```python
from build123d import *

# Parameters (mm, degrees)
F1_DEPTH     = 6
F2_C1_SIZE2  = 3
F2_C1_SIZE   = 1.7320508076
F2_C2_SIZE2  = 3
F2_C2_SIZE   = 1.7320508076
F2_C3_SIZE2  = 1.7320508076
F2_C3_SIZE   = 3
F2_C4_SIZE2  = 3
F2_C4_SIZE   = 1.7320508076
F2_C5_SIZE2  = 1.7320508076
F2_C5_SIZE   = 3
F2_C6_SIZE2  = 3
F2_C6_SIZE   = 1.7320508076
F2_C7_SIZE2  = 1.7320508076
F2_C7_SIZE   = 3
F2_C8_SIZE2  = 3
F2_C8_SIZE   = 1.7320508076
F2_C9_SIZE2  = 1.7320508076
F2_C9_SIZE   = 3
F2_C10_SIZE2 = 3
F2_C10_SIZE  = 1.7320508076
F2_C11_SIZE2 = 3
F2_C11_SIZE  = 1.7320508076
F2_C12_SIZE2 = 3
F2_C12_SIZE  = 1.7320508076
F2_C13_SIZE2 = 1.7320508076
F2_C13_SIZE  = 3
F2_C14_SIZE2 = 3
F2_C14_SIZE  = 1.7320508076
F2_C15_SIZE2 = 3
F2_C15_SIZE  = 1.7320508076
F2_C16_SIZE2 = 3
F2_C16_SIZE  = 1.7320508076
F2_C17_SIZE2 = 1.7320508076
F2_C17_SIZE  = 3
F2_C18_SIZE2 = 3
F2_C18_SIZE  = 1.7320508076
F2_C19_SIZE2 = 3
F2_C19_SIZE  = 1.7320508076
F2_C20_SIZE2 = 3
F2_C20_SIZE  = 1.7320508076
F2_C21_SIZE2 = 1.7320508076
F2_C21_SIZE  = 3
F2_C22_SIZE2 = 3
F2_C22_SIZE  = 1.7320508076
F2_C23_SIZE2 = 3
F2_C23_SIZE  = 1.7320508076
F2_C24_SIZE2 = 3
F2_C24_SIZE  = 1.7320508076
F3_R         = 1


with BuildPart() as f1:
    # F0 (on Top) → F1 (new body)
    with BuildSketch(Plane.XY):
        with BuildLine():
            ThreePointArc((5.4975, 9.5219493146), (9.5219493146, 5.4975), (10.995, 0))
            Line((10.995, 0), (14.995, 0))
            ThreePointArc((14.995, 0), (17.8875950663, 4.5341861944), (23.2185377782, 3.8221465425))
            Line((23.2185377782, 3.8221465425), (38.9711431703, 22.5))
            Line((38.9711431703, 22.5), (14.9193448919, 18.1967702834))
            ThreePointArc((14.9193448919, 18.1967702834), (12.870517963, 13.2240186428), (7.4975, 12.9860509297))
            Line((7.4975, 12.9860509297), (5.4975, 9.5219493146))
        make_face()
        with BuildLine():
            ThreePointArc((-5.4975, 9.5219493146), (0, 10.995), (5.4975, 9.5219493146))
            Line((5.4975, 9.5219493146), (7.4975, 12.9860509297))
            ThreePointArc((7.4975, 12.9860509297), (5.0170771033, 17.7582048372), (8.2991928863, 22.0189168259))
            Line((8.2991928863, 22.0189168259), (0, 45))
            Line((0, 45), (-8.2991928863, 22.0189168259))
            ThreePointArc((-8.2991928863, 22.0189168259), (-5.0170771033, 17.7582048372), (-7.4975, 12.9860509297))
            Line((-7.4975, 12.9860509297), (-5.4975, 9.5219493146))
        make_face()
        with BuildLine():
            ThreePointArc((-10.995, 0), (-9.5219493146, 5.4975), (-5.4975, 9.5219493146))
            Line((-5.4975, 9.5219493146), (-7.4975, 12.9860509297))
            ThreePointArc((-7.4975, 12.9860509297), (-12.870517963, 13.2240186428), (-14.9193448919, 18.1967702834))
            Line((-14.9193448919, 18.1967702834), (-38.9711431703, 22.5))
            Line((-38.9711431703, 22.5), (-23.2185377782, 3.8221465425))
            ThreePointArc((-23.2185377782, 3.8221465425), (-17.8875950663, 4.5341861944), (-14.995, 0))
            Line((-14.995, 0), (-10.995, 0))
        make_face()
        with BuildLine():
            Line((-7.4975, -12.9860509297), (-5.4975, -9.5219493146))
            ThreePointArc((-5.4975, -9.5219493146), (-9.5219493146, -5.4975), (-10.995, 0))
            Line((-10.995, 0), (-14.995, 0))
            ThreePointArc((-14.995, 0), (-17.8875950663, -4.5341861944), (-23.2185377782, -3.8221465425))
            Line((-23.2185377782, -3.8221465425), (-38.9711431703, -22.5))
            Line((-38.9711431703, -22.5), (-14.9193448919, -18.1967702834))
            ThreePointArc((-14.9193448919, -18.1967702834), (-12.870517963, -13.2240186428), (-7.4975, -12.9860509297))
        make_face()
        with BuildLine():
            Line((7.4975, -12.9860509297), (5.4975, -9.5219493146))
            ThreePointArc((5.4975, -9.5219493146), (0, -10.995), (-5.4975, -9.5219493146))
            Line((-5.4975, -9.5219493146), (-7.4975, -12.9860509297))
            ThreePointArc((-7.4975, -12.9860509297), (-5.0170771033, -17.7582048372), (-8.2991928863, -22.0189168259))
            Line((-8.2991928863, -22.0189168259), (0, -45))
            Line((0, -45), (8.2991928863, -22.0189168259))
            ThreePointArc((8.2991928863, -22.0189168259), (5.0170771033, -17.7582048372), (7.4975, -12.9860509297))
        make_face()
        with BuildLine():
            Line((14.995, 0), (10.995, 0))
            ThreePointArc((10.995, 0), (9.5219493146, -5.4975), (5.4975, -9.5219493146))
            Line((5.4975, -9.5219493146), (7.4975, -12.9860509297))
            ThreePointArc((7.4975, -12.9860509297), (12.870517963, -13.2240186428), (14.9193448919, -18.1967702834))
            Line((14.9193448919, -18.1967702834), (38.9711431703, -22.5))
            Line((38.9711431703, -22.5), (23.2185377782, -3.8221465425))
            ThreePointArc((23.2185377782, -3.8221465425), (17.8875950663, -4.5341861944), (14.995, 0))
        make_face()
    extrude(amount=F1_DEPTH)

    # F2: chamfer of 3 x 1.7320508076 on 24 edges, made by hand

    # F2_c1
    f2_c1_edges = [f1.edges().sort_by_distance(p)[0] for p in [
        (31.0948404742, 13.1610732713, 0),
    ]]
    f2_c1_side = f1.faces().sort_by_distance((31.0948404742, 13.1610732713, 0.0346410162))[0]
    chamfer(f2_c1_edges, length=F2_C1_SIZE, length2=F2_C1_SIZE2, reference=f2_c1_side)

    # F2_c2
    f2_c2_edges = [f1.edges().sort_by_distance(p)[0] for p in [
        (31.0948404742, 13.1610732713, 6),
    ]]
    f2_c2_side = f1.faces().sort_by_distance((31.0948404742, 13.1610732713, 5.9653589838))[0]
    chamfer(f2_c2_edges, length=F2_C2_SIZE, length2=F2_C2_SIZE2, reference=f2_c2_side)

    # F2_c3
    f2_c3_edges = [f1.edges().sort_by_distance(p)[0] for p in [
        (24.6342857936, 19.9349198346, 0),
    ]]
    f2_c3_side = f1.faces().sort_by_distance((24.6342857936, 19.9349198346, 0.0346410162))[0]
    chamfer(f2_c3_edges, length=F2_C3_SIZE, length2=F2_C3_SIZE2, reference=f2_c3_side)

    # F2_c4
    f2_c4_edges = [f1.edges().sort_by_distance(p)[0] for p in [
        (24.6342857936, 19.9349198346, 6),
    ]]
    f2_c4_side = f1.faces().sort_by_distance((24.6342857936, 19.9349198346, 5.9653589838))[0]
    chamfer(f2_c4_edges, length=F2_C4_SIZE, length2=F2_C4_SIZE2, reference=f2_c4_side)

    # F2_c5
    f2_c5_edges = [f1.edges().sort_by_distance(p)[0] for p in [
        (4.1495964431, 33.509458413, 0),
    ]]
    f2_c5_side = f1.faces().sort_by_distance((4.1170149125, 33.4976921961, 0))[0]
    chamfer(f2_c5_edges, length=F2_C5_SIZE, length2=F2_C5_SIZE2, reference=f2_c5_side)

    # F2_c6
    f2_c6_edges = [f1.edges().sort_by_distance(p)[0] for p in [
        (4.1495964431, 33.509458413, 6),
    ]]
    f2_c6_side = f1.faces().sort_by_distance((4.1495964431, 33.509458413, 5.9653589838))[0]
    chamfer(f2_c6_edges, length=F2_C6_SIZE, length2=F2_C6_SIZE2, reference=f2_c6_side)

    # F2_c7
    f2_c7_edges = [f1.edges().sort_by_distance(p)[0] for p in [
        (-4.9470041023, 31.3013772186, 0),
    ]]
    f2_c7_side = f1.faces().sort_by_distance((-4.9144225717, 31.2896110018, 0))[0]
    chamfer(f2_c7_edges, length=F2_C7_SIZE, length2=F2_C7_SIZE2, reference=f2_c7_side)

    # F2_c8
    f2_c8_edges = [f1.edges().sort_by_distance(p)[0] for p in [
        (-4.9470041023, 31.3013772186, 6),
    ]]
    f2_c8_side = f1.faces().sort_by_distance((-4.9470041023, 31.3013772186, 5.9653589838))[0]
    chamfer(f2_c8_edges, length=F2_C8_SIZE, length2=F2_C8_SIZE2, reference=f2_c8_side)

    # F2_c9
    f2_c9_edges = [f1.edges().sort_by_distance(p)[0] for p in [
        (-26.9452440311, 20.3483851417, 0),
    ]]
    f2_c9_side = f1.faces().sort_by_distance((-26.9513449538, 20.3142856, 0))[0]
    chamfer(f2_c9_edges, length=F2_C9_SIZE, length2=F2_C9_SIZE2, reference=f2_c9_side)

    # F2_c10
    f2_c10_edges = [f1.edges().sort_by_distance(p)[0] for p in [
        (-26.9452440311, 20.3483851417, 6),
    ]]
    f2_c10_side = f1.faces().sort_by_distance((-26.9452440311, 20.3483851417, 5.9653589838))[0]
    chamfer(f2_c10_edges, length=F2_C10_SIZE, length2=F2_C10_SIZE2, reference=f2_c10_side)

    # F2_c11
    f2_c11_edges = [f1.edges().sort_by_distance(p)[0] for p in [
        (-29.581289896, 11.3664573841, 0),
    ]]
    f2_c11_side = f1.faces().sort_by_distance((-29.5548092879, 11.3887907089, 0))[0]
    chamfer(f2_c11_edges, length=F2_C11_SIZE, length2=F2_C11_SIZE2, reference=f2_c11_side)

    # F2_c12
    f2_c12_edges = [f1.edges().sort_by_distance(p)[0] for p in [
        (-29.581289896, 11.3664573841, 6),
    ]]
    f2_c12_side = f1.faces().sort_by_distance((-29.581289896, 11.3664573841, 5.9653589838))[0]
    chamfer(f2_c12_edges, length=F2_C12_SIZE, length2=F2_C12_SIZE2, reference=f2_c12_side)

    # F2_c13
    f2_c13_edges = [f1.edges().sort_by_distance(p)[0] for p in [
        (-31.0948404742, -13.1610732713, 0),
    ]]
    f2_c13_side = f1.faces().sort_by_distance((-31.0683598662, -13.1834065961, 0))[0]
    chamfer(f2_c13_edges, length=F2_C13_SIZE, length2=F2_C13_SIZE2, reference=f2_c13_side)

    # F2_c14
    f2_c14_edges = [f1.edges().sort_by_distance(p)[0] for p in [
        (-31.0948404742, -13.1610732713, 6),
    ]]
    f2_c14_side = f1.faces().sort_by_distance((-31.0948404742, -13.1610732713, 5.9653589838))[0]
    chamfer(f2_c14_edges, length=F2_C14_SIZE, length2=F2_C14_SIZE2, reference=f2_c14_side)

    # F2_c15
    f2_c15_edges = [f1.edges().sort_by_distance(p)[0] for p in [
        (-24.6342857936, -19.9349198346, 0),
    ]]
    f2_c15_side = f1.faces().sort_by_distance((-24.6403867163, -19.9008202929, 0))[0]
    chamfer(f2_c15_edges, length=F2_C15_SIZE, length2=F2_C15_SIZE2, reference=f2_c15_side)

    # F2_c16
    f2_c16_edges = [f1.edges().sort_by_distance(p)[0] for p in [
        (-24.6342857936, -19.9349198346, 6),
    ]]
    f2_c16_side = f1.faces().sort_by_distance((-24.6342857936, -19.9349198346, 5.9653589838))[0]
    chamfer(f2_c16_edges, length=F2_C16_SIZE, length2=F2_C16_SIZE2, reference=f2_c16_side)

    # F2_c17
    f2_c17_edges = [f1.edges().sort_by_distance(p)[0] for p in [
        (-4.1495964431, -33.509458413, 0),
    ]]
    f2_c17_side = f1.faces().sort_by_distance((-4.1170149125, -33.4976921961, 0))[0]
    chamfer(f2_c17_edges, length=F2_C17_SIZE, length2=F2_C17_SIZE2, reference=f2_c17_side)

    # F2_c18
    f2_c18_edges = [f1.edges().sort_by_distance(p)[0] for p in [
        (-4.1495964431, -33.509458413, 6),
    ]]
    f2_c18_side = f1.faces().sort_by_distance((-4.1495964431, -33.509458413, 5.9653589838))[0]
    chamfer(f2_c18_edges, length=F2_C18_SIZE, length2=F2_C18_SIZE2, reference=f2_c18_side)

    # F2_c19
    f2_c19_edges = [f1.edges().sort_by_distance(p)[0] for p in [
        (4.9470041023, -31.3013772186, 0),
    ]]
    f2_c19_side = f1.faces().sort_by_distance((4.9144225717, -31.2896110018, 0))[0]
    chamfer(f2_c19_edges, length=F2_C19_SIZE, length2=F2_C19_SIZE2, reference=f2_c19_side)

    # F2_c20
    f2_c20_edges = [f1.edges().sort_by_distance(p)[0] for p in [
        (4.9470041023, -31.3013772186, 6),
    ]]
    f2_c20_side = f1.faces().sort_by_distance((4.9470041023, -31.3013772186, 5.9653589838))[0]
    chamfer(f2_c20_edges, length=F2_C20_SIZE, length2=F2_C20_SIZE2, reference=f2_c20_side)

    # F2_c21
    f2_c21_edges = [f1.edges().sort_by_distance(p)[0] for p in [
        (26.9452440311, -20.3483851417, 0),
    ]]
    f2_c21_side = f1.faces().sort_by_distance((26.9513449538, -20.3142856, 0))[0]
    chamfer(f2_c21_edges, length=F2_C21_SIZE, length2=F2_C21_SIZE2, reference=f2_c21_side)

    # F2_c22
    f2_c22_edges = [f1.edges().sort_by_distance(p)[0] for p in [
        (26.9452440311, -20.3483851417, 6),
    ]]
    f2_c22_side = f1.faces().sort_by_distance((26.9452440311, -20.3483851417, 5.9653589838))[0]
    chamfer(f2_c22_edges, length=F2_C22_SIZE, length2=F2_C22_SIZE2, reference=f2_c22_side)

    # F2_c23
    f2_c23_edges = [f1.edges().sort_by_distance(p)[0] for p in [
        (29.581289896, -11.3664573841, 0),
    ]]
    f2_c23_side = f1.faces().sort_by_distance((29.5548092879, -11.3887907089, 0))[0]
    chamfer(f2_c23_edges, length=F2_C23_SIZE, length2=F2_C23_SIZE2, reference=f2_c23_side)

    # F2_c24
    f2_c24_edges = [f1.edges().sort_by_distance(p)[0] for p in [
        (29.581289896, -11.3664573841, 6),
    ]]
    f2_c24_side = f1.faces().sort_by_distance((29.581289896, -11.3664573841, 5.9653589838))[0]
    chamfer(f2_c24_edges, length=F2_C24_SIZE, length2=F2_C24_SIZE2, reference=f2_c24_side)

    # F3
    f3_edges = [f1.edges().sort_by_distance(p)[0] for p in [
        (-10.995, 0, 0),
        (-10.995, 0, 6),
    ]]
    fillet(f3_edges, radius=F3_R)


solid = f1.part
```
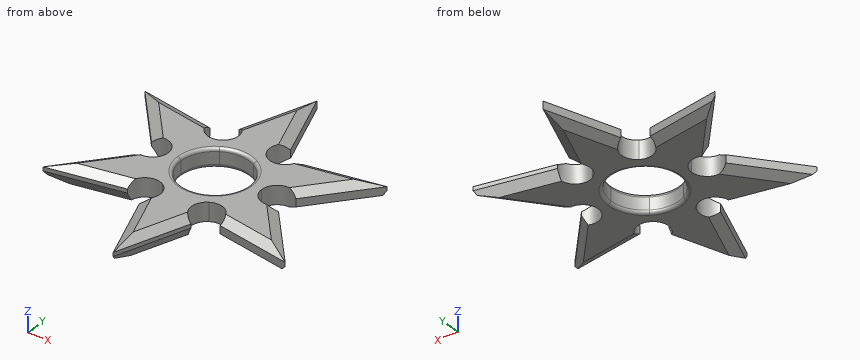
Verification items for the finished model (mm, model axes). Give positions to 0.01 mm unless a question says otherwise; leave off trailing zeros. Write each loop counter-clockwise with the first axis right and the second up, starting at its lowest first coordinate (ties: lowest second). Pieces come first, ordered by that corner, then holes. Notation, with made-up numbers: (31, -15.5) - (51, -15.5) arc R31 cw to (51, 22.5) - close; hole circle Ø7 at (-22, -2). An arc over 180 degrees is marked (long way). Put each result on its own line as item: value.
Q1. Scan lines: probe 1 along X at (y, z) = (-17.5, 2.5); probe 2 along X at (y, z) = (4, 2) (3 decimals); probe 3 along Y at (x, z) = (25, 2.25). Record each from-to range of solid material in increasing order. Write a range as from..to.
Result:
probe 1: -34.75..-14.99, -5..5, 14.99..34.38
probe 2: -16.995..-10.242, 10.242..16.995, 22.995..23.369
probe 3: -20..-6.61, 5.93..19.56
Q2. Section check C-C on x = 16.5. Record the cut outline in (y, z).
Result:
outline: (-18.48, 1.73) - (-15.43, 0) - (-3.58, 0) - (-3.58, 6) - (-15.43, 6) - (-18.48, 4.27) - close; (3.58, 0) - (16.72, 0) - (18.48, 3) - (18.48, 4.27) - (15.43, 6) - (3.58, 6) - close
Q3. Section check B-B on y = -29. Record the cut outline in (x, z).
Result:
outline: (-5.78, 1.73) - (-2.59, 0) - (3.94, 0) - (5.78, 3) - (5.78, 4.27) - (2.59, 6) - (-2.59, 6) - (-5.78, 4.27) - close
Q4. Depth check by flat-ended pin: P1, Ø1, axis at x = 26.5, z = 5.5, coming from the -Y side; P2, Ø3, axis at y = 26.5, z = 3, coming from the -X side. Enter the tip coordinate at first touch or a pass-through.
Result:
P1: y = -18.99
P2: x = -7.22
Q5. Section check A-A on x = -28. Record the cut outline in (y, z), and give its area (3 significant figures).
Result:
outline: (-20.54, 3) - (-18.78, 0) - (-14.14, 0) - (-9.49, 1.73) - (-9.49, 4.27) - (-14.14, 6) - (-17.49, 6) - (-20.54, 4.27) - close; (9.49, 3) - (12.18, 0) - (17.49, 0) - (20.54, 1.73) - (20.54, 4.27) - (17.49, 6) - (14.14, 6) - (9.49, 4.27) - close
area: 106 mm2
Q6. Section check D-D on y = 35. Record the cut outline in (x, z).
Result:
outline: (-3.61, 1.73) - (-0.42, 0) - (0.42, 0) - (3.61, 1.73) - (3.61, 4.27) - (0.42, 6) - (-0.42, 6) - (-3.61, 4.27) - close
